Verification items for the finished model (mm, model axes). Face numbers are marked on the shaded views. Coordinates: 2 decimals unless noted, no trailing zeros. Loops run counter-clockwise (first coordinate to the right, second up) from the corner with the lowest first, then second, coordinate; pieces in that order, holes last. Notation, with made-up numbers: (45.5, -31.5) - (88.5, -31.5) arc R10 ccw to (88.5, -20.5) - close; hole circle Ø10 at (52, 10.5). An arc over 180 degrees is marked (long way). One line per item, written item: value. Start each with the question number.
(1) Section check C-C (z = -4.5). Record the boundary of the cut face in (x, y).
(2) Draft check along Z on the marked faces 1 and 2. Enter one of: +Z half, -Z half, draft (parallel to the pull), parting line (faces both ways), or undercut.
(3) Section check B-B (x = 7.62). Record the boundary of the cut face in (y, z), plus the area to 3 significant figures.
(4) Section check D-D (x = 25.4). Record the boundary of the cut face in (y, z).
(5) Thickness scan on probe 1 along X at (y, z) = (7.5, -1); probe 2 along Z at (x, y) = (19.5, 36.5); probe 3 along X at (y, z) = (2.5, -4.5). Record the ranges inside material, lowest first. Write a range as [from, to].
(6) Gauge pin test, flat ends, axial feed: P1, Ø12, axis at x = 9.5, y = 23.5, coming from the -Z side; P2, Ø4, axis at x = 17, y = 30.5, coming from the +Z side; P3, Ø4.5, axis at x = 25.4, z = -2.86, coming from the -Y side; P4, Ø2, axis at y = 17, z = -1.5, coming from the +X side. Record the tip position at first contact, or that the pin passes through.
(7) Section check A-A (y = 43.18). Record the boundary of the cut face in (x, z) (1 decimal).
```python
from build123d import *

# Parameters (mm, degrees)
SKETCH1_W           = 20.32
SKETCH1_H           = 2.032
SKETCH1_R           = 4.445
BOSS_EXTRUDE1_DEPTH = 50.8
SKETCH2_R           = 2.54
CUT_EXTRUDE1_DEPTH  = 50.8
CUT_EXTRUDE2_START  = 8.89
SKETCH1_3_R         = 4.445
CUT_EXTRUDE2_DEPTH  = 11.43
CUT_EXTRUDE3_START  = 30.48
SKETCH1_5_R         = 4.445
CUT_EXTRUDE3_DEPTH  = 11.43
SKETCH3_R           = 2.54
CUT_EXTRUDE4_DEPTH  = 60.369104181


with BuildPart() as part:
    # Sketch1 → Boss-Extrude1 (new body)
    with BuildSketch(Plane(origin=(0, 0, 0), x_dir=(1, 0, 0), z_dir=(0, 1, 0))):
        with Locations((10.16, 1.016)):
            Rectangle(SKETCH1_W, SKETCH1_H)
        with BuildLine():
            Line((21.032326163, 2.032), (20.32, 2.032))
            Line((20.32, 2.032), (20.32, 0))
            Line((20.32, 0), (21.995191819, 0))
            ThreePointArc((21.995191819, 0), (21.383144864, 0.954108338), (21.032326163, 2.032))
        make_face()
        with Locations((25.4, 2.8575)):
            Circle(SKETCH1_R)
    extrude(amount=BOSS_EXTRUDE1_DEPTH)

    # Sketch2 → Cut-Extrude1 (cut)
    with BuildSketch(Plane(origin=(0, 0, -2.032), x_dir=(-1, 0, 0), z_dir=(0, 0, -1))):
        with Locations((-7.62, 43.18)):
            Circle(SKETCH2_R)
        with Locations((-7.62, 7.62)):
            Circle(SKETCH2_R)
    extrude(amount=-CUT_EXTRUDE1_DEPTH, mode=Mode.SUBTRACT)

    # Sketch1_3 → Cut-Extrude2 (cut)
    with BuildSketch(Plane(origin=(0, 0, 0), x_dir=(1, 0, 0), z_dir=(0, 1, 0)).offset(CUT_EXTRUDE2_START)):
        with BuildLine():
            Line((21.032326163, 2.032), (20.32, 2.032))
            Line((20.32, 2.032), (20.32, 0))
            Line((20.32, 0), (21.995191819, 0))
            ThreePointArc((21.995191819, 0), (21.383144864, 0.954108338), (21.032326163, 2.032))
        make_face()
        with Locations((25.4, 2.8575)):
            Circle(SKETCH1_3_R)
    extrude(amount=CUT_EXTRUDE2_DEPTH, mode=Mode.SUBTRACT)

    # Sketch1_5 → Cut-Extrude3 (cut)
    with BuildSketch(Plane(origin=(0, 0, 0), x_dir=(1, 0, 0), z_dir=(0, 1, 0)).offset(CUT_EXTRUDE3_START)):
        with Locations((25.4, 2.8575)):
            Circle(SKETCH1_5_R)
        with BuildLine():
            Line((21.032326163, 2.032), (20.32, 2.032))
            Line((20.32, 2.032), (20.32, 0))
            Line((20.32, 0), (21.995191819, 0))
            ThreePointArc((21.995191819, 0), (21.383144864, 0.954108338), (21.032326163, 2.032))
        make_face()
    extrude(amount=CUT_EXTRUDE3_DEPTH, mode=Mode.SUBTRACT)

    # Sketch3 → Cut-Extrude4 (cut, through all)
    with BuildSketch(Plane(origin=(0, 50.8, 0), x_dir=(1, 0, 0), z_dir=(0, 1, 0))):
        with Locations(Location((25.4, 2.8575, 0), (0, 0, 270))):
            Circle(SKETCH3_R)
    extrude(amount=-CUT_EXTRUDE4_DEPTH, mode=Mode.SUBTRACT)


solid = part.part
```
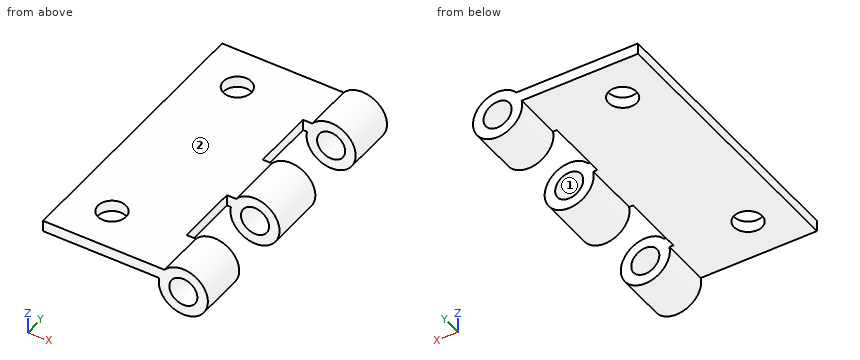
Responses:
1. outline: (21.27, 0) - (23.46, 0) - (23.46, 8.89) - (21.27, 8.89) - close; (21.27, 20.32) - (23.46, 20.32) - (23.46, 30.48) - (21.27, 30.48) - close; (21.27, 41.91) - (23.46, 41.91) - (23.46, 50.8) - (21.27, 50.8) - close; (27.34, 0) - (29.53, 0) - (29.53, 8.89) - (27.34, 8.89) - close; (27.34, 20.32) - (29.53, 20.32) - (29.53, 30.48) - (27.34, 30.48) - close; (27.34, 41.91) - (29.53, 41.91) - (29.53, 50.8) - (27.34, 50.8) - close
2. face 1: undercut
2. face 2: +Z half
3. outline: (0, -2.03) - (5.08, -2.03) - (5.08, 0) - (0, 0) - close; (10.16, -2.03) - (40.64, -2.03) - (40.64, 0) - (10.16, 0) - close; (45.72, -2.03) - (50.8, -2.03) - (50.8, 0) - (45.72, 0) - close
3. area: 82.6 mm²
4. outline: (0, -7.3) - (8.89, -7.3) - (8.89, -5.4) - (0, -5.4) - close; (0, -0.32) - (8.89, -0.32) - (8.89, 1.59) - (0, 1.59) - close; (20.32, -7.3) - (30.48, -7.3) - (30.48, -5.4) - (20.32, -5.4) - close; (20.32, -0.32) - (30.48, -0.32) - (30.48, 1.59) - (20.32, 1.59) - close; (41.91, -7.3) - (50.8, -7.3) - (50.8, -5.4) - (41.91, -5.4) - close; (41.91, -0.32) - (50.8, -0.32) - (50.8, 1.59) - (41.91, 1.59) - close
5. probe 1: x = [0, 5.08], [10.16, 23.67], [27.13, 29.44]
5. probe 2: z = [-2.03, 0]
5. probe 3: x = [21.27, 23.46], [27.34, 29.53]
6. P1: stops at z = -2.03
6. P2: stops at z = 0
6. P3: passes through
6. P4: stops at x = 20.32
7. outline: (0, -2) - (5.1, -2) - (5.1, 0) - (0, 0) - close; (10.2, -2) - (21, -2) arc R4.4 ccw (long way) to (22, 0) - (10.2, 0) - close; hole circle Ø5.1 at (25.4, -2.9)
